Can you work these out from the model? Positions are in its coordinate system, mm. A direction names the side the tool comes from. Coordinates: 2 decimals unless noted, no trailing zeros. Order: outer loops, then holes, each group sorted by start corner. A loop starts at its lowest first (then second) coordinate and runs counter-clockwise, first axis right, second up. Notation, with made-up numbers: M 78.25,24 L 121.25,24 A21 ccw 121.25,63 Z; hole C -14.75,-2 d7. An arc over 180 degrees is marked long. Answer as a JSON object with one key per item and string values.
Autodesk Inventor part; units mm, degrees
ref_plane "YZ Plane" through (0, 0, 0) normal (1, 0, 0) x (0, 1, 0)
ref_plane "XZ Plane" through (0, 0, 0) normal (0, 1, 0) x (-1, 0, 0)
ref_plane "XY Plane" through (0, 0, 0) normal (0, 0, 1) x (1, 0, 0)
sketch "Sketch6" plane through (0, 0, 0) normal (0, 0, 1) x (1, 0, 0)
  circle A0 centre (0, 0) radius 12.5
  dimension "d29" = 25
extrude "base" add sketch "Sketch6" along normal blind 9
sketch "Sketch8" plane through (0, 0, 9) normal (0, 0, 1) x (1, 0, 0)
  circle A0 centre (0, 0) radius 9.4
  dimension "d39" = 18.8
extrude "Extrusion8" cut sketch "Sketch8" against normal blind 8
sketch "Sketch7" plane through (0, 0, 9) normal (0, 0, 1) x (1, 0, 0)
  line L0 (0, 0) -> (0, 9)
  circle A0 centre (0, 9) radius 2
  dimension "d33" = 9
  dimension "d34" = 4
extrude "ball_place" cut sketch "Sketch7" against normal blind 8
fillet "Fillet5" radius 8 2 edges at (-1.9913, 9.1867, 5) (1.9913, 9.1867, 5)
pattern_circular "Circular Pattern2" count 6 over 360 about axis through (0, 0, 9) along (0, 0, -1) of "ball_place", "Fillet5"
equation "\"BendRadius\" = Thickness"
equation "\"BendReliefWidth\" = Thickness"
equation "\"BendReliefDepth\" = 0.5 * Thickness"
equation "\"CornerReliefSize\" = 4 * Thickness"
equation "\"MinimumRemnant\" = 2 * Thickness"
equation "\"TransitionRadius\" = BendRadius"
equation "\"JacobiRadiusSize\" = BendRadius"
equation "\"GapSize\" = Thickness"
properties part number "embrague_1"
Item 1: I want a section at B-B, the plane x = 0. Write out the boundary of the cut face in (y, z).
Answers follow:
{"outline": "M -12.5,0 L 12.5,0 L 12.5,9 L 11,9 L 11,1 L -11,1 L -11,9 L -12.5,9 Z"}
Item 2: I'm going to push flat-ended pins straight in: pin 1 (5 mm diameter, centred on x = -4, z = 1.5, fed in from +Y); pin 2 (2 mm diameter, centred on x = -7, z = 7.5, fed in from -Y); pin 3 (1 mm diameter, centred on y = 6.5, z = 6.5, fed in from +X). Where does each tip first touch, or does it pass through?
Answers follow:
{"pin 1": "stops at y = 12.41", "pin 2": "stops at y = -10.97", "pin 3": "stops at x = 10.97"}
Item 3: I want a section at A-A, the plane y = 0. Write out the boundary of the cut face in (x, z).
Answers follow:
{"outline": "M -12.5,0 L 12.5,0 L 12.5,9 L 9.4,9 L 9.4,1 L -9.4,1 L -9.4,9 L -12.5,9 Z"}
Item 4: If we mould it in two halves opening along X, with no side actions, what happens to faces 1 (the flat face through (0, 0, 0)), 2 (the cylindrical face through (4.69, -8.146, 5.056)), 3 (the cylindrical face through (-4.69, 8.146, 5.056)), 4 (the cylindrical face through (11.923, -3.755, 4.437))? For each: pulls with the +X half, pulls with the -X half, needs draft (parallel to the pull), parting line crosses it, or undercut.
Answers follow:
{"face 1": "needs draft", "face 2": "undercut", "face 3": "undercut", "face 4": "parting line crosses it"}
Item 5: Which directions (+Z, -Z, +X, -X, +Y, -Y) give clear straight access to the entire face, cutting with the end or side of a thin tool? Please do faces 5 (the flat face through (0, 0, 1)), 6 (the flat face through (6.4, -7.3, 9)).
Answers follow:
{"face 5": "+Z", "face 6": "+Z, +X, -X, +Y, -Y"}
Item 6: Please list where these lines run through material, in increasing order: line 1 (Z direction, x = 6.5, y = -4); line 2 (X direction, y = 5.25, z = 3.5); line 3 (Y direction, x = -7.25, z = 6.25).
Answers follow:
{"line 1": "z = 0 to 1", "line 2": "x = -11.34 to -9.65, 9.65 to 11.34", "line 3": "y = -10.18 to -6.74, 6.74 to 10.18"}
